Verification items for this drawing (mm, ordinates from the low corner). A direction names the side the tool comes from. Give positions to 0.01 mm unless a question says otherwise; leave off trailing zeros. Order: outer loops, then holes, each group sorted by start corner. A loop starts at its lowest first (then second) coordinate and runs counter-clockwise, first axis right, second up.
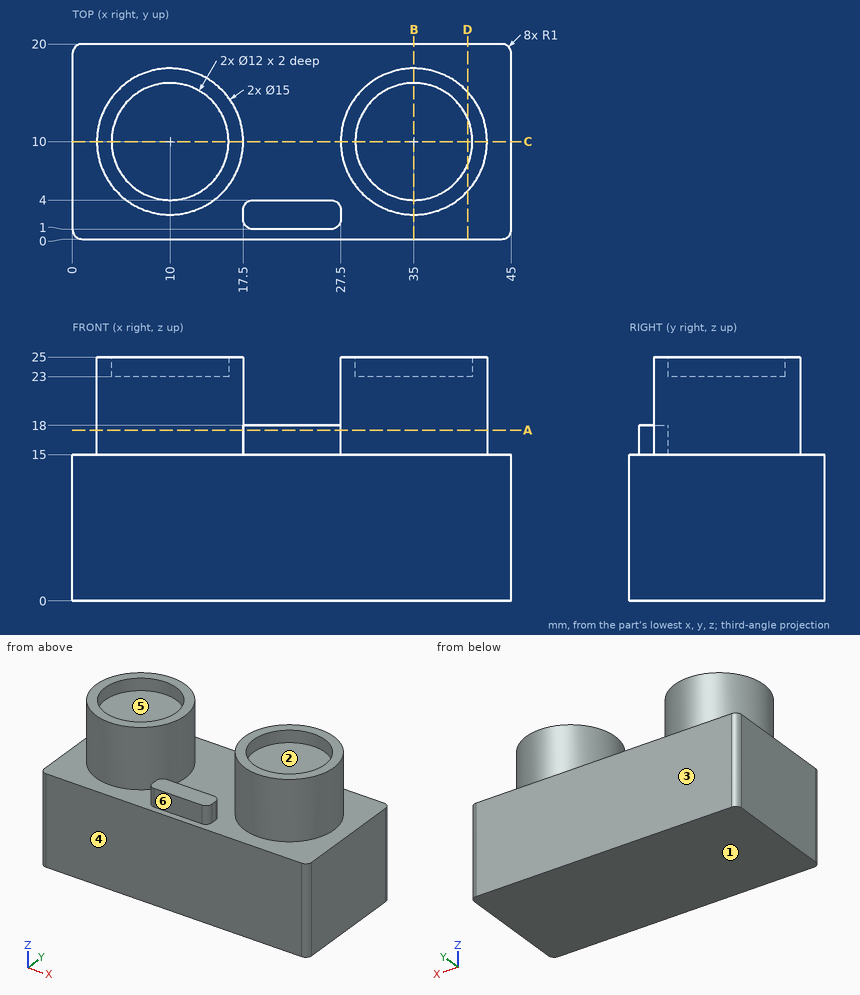
Q1. Cross-section at A-A, the plane z = 17.5. Record the boundary of the cut face in (x, y), and give its area (3 significant figures).
Q2. Thickness scan on L1, parallel to Y at x = 10, z = 23.7; L2, parallel to Z at x = 43.5, y = 6.5; L3, parallel to Z at x = 39, y = 6. Record the ranges inside material, lowest first.
Q3. Access from +Z, -Z, +X, -X, +Y, -Y to the whole of each face (thin tool, end or side, straight path). Record for the marked faces 4, 5 and 6.
Q4. Cross-section at D-D, the plane x = 40.5. Record the boundary of the cut face in (y, z).
Q5. Release check for a two-part mould opening along Y. For the marked faces 1, 2 and 3 record: pulls with the +Y half, pulls with the -Y half, needs draft (parallel to the pull), parting line crosses it, or undercut.
Q6. Cross-section at C-C, the plane y = 10. Record the boundary of the cut face in (x, z), and give its area (3 significant figures).
Q7. Cross-section at B-B, the plane x = 35. Record the boundary of the cut face in (y, z), and give its area (3 significant figures).
Q8. Gauge pin test, flat ends, axial feed: P1, Ø9.5, axis at x = 35, y = 10, coming from the +Z side; P2, Ø3.5, axis at x = 24, z = 16, coming from the +Y side; P3, Ø2.5, axis at x = 21, y = 2, coming from the +Z side; P4, Ø1, axis at x = 30, z = 16.5, coming from the -Y side. Record the tip position at first contact, or that the pin passes through.
Answers follow:
1. outline: circle Ø15 at (10, 10); (17.5, 2) arc R1 ccw to (18.5, 1) - (26.5, 1) arc R1 ccw to (27.5, 2) - (27.5, 3) arc R1 ccw to (26.5, 4) - (18.5, 4) arc R1 ccw to (17.5, 3) - close; circle Ø15 at (35, 10)
1. area: 383 mm2
2. L1: y = 2.5 to 4, 16 to 17.5
2. L2: z = 0 to 15
2. L3: z = 0 to 23
3. face 4: +Z, -Z, +X, -X, -Y
3. face 5: +Z
3. face 6: +Z, +X, -X, -Y
4. outline: (0, 0) - (20, 0) - (20, 15) - (15.1, 15) - (15.1, 25) - (12.4, 25) - (12.4, 23) - (7.6, 23) - (7.6, 25) - (4.9, 25) - (4.9, 15) - (0, 15) - close
5. face 1: needs draft
5. face 2: undercut
5. face 3: pulls with the +Y half
6. outline: (0, 0) - (45, 0) - (45, 15) - (42.5, 15) - (42.5, 25) - (41, 25) - (41, 23) - (29, 23) - (29, 25) - (27.5, 25) - (27.5, 15) - (17.5, 15) - (17.5, 25) - (16, 25) - (16, 23) - (4, 23) - (4, 25) - (2.5, 25) - (2.5, 15) - (0, 15) - close
6. area: 927 mm2
7. outline: (0, 0) - (20, 0) - (20, 15) - (17.5, 15) - (17.5, 25) - (16, 25) - (16, 23) - (4, 23) - (4, 25) - (2.5, 25) - (2.5, 15) - (0, 15) - close
7. area: 426 mm2
8. P1: stops at z = 23
8. P2: stops at y = 20
8. P3: stops at z = 18
8. P4: stops at y = 4
